For this review, take the finished solid that the model builds, in its own axes (mm). A direction names the side the tool comes from. Round coordinates to 2 decimals unless told otherwise and drop trailing zeros. Loops run counter-clockwise (first coordinate to the right, second up) from the corner with the lowest first, then second, coordinate; pieces in that order, holes last.
```python
from build123d import *

# Parameters (mm, degrees)
F1_DEPTH = 5
F2_T     = -2.5
F3_DEPTH = 25


with BuildPart() as f1:
    # F0 (on Front) → F1 (new body)
    with BuildSketch(Plane.XZ):
        with BuildLine():
            Line((-32.5, -5), (32.5, -5))
            ThreePointArc((32.5, -5), (36.0355339059, -3.5355339059), (37.5, 0))
            ThreePointArc((37.5, 0), (36.0355339059, 3.5355339059), (32.5, 5))
            Line((32.5, 5), (-32.5, 5))
            ThreePointArc((-32.5, 5), (-36.0355339059, 3.5355339059), (-37.5, 0))
            ThreePointArc((-37.5, 0), (-36.0355339059, -3.5355339059), (-32.5, -5))
        make_face()
    extrude(amount=F1_DEPTH)

    # F2
    f2_openings = [f1.faces().sort_by_distance(p)[0] for p in [
        (0, -5, 0),
    ]]
    offset(amount=F2_T, openings=f2_openings)

    # F3 (cut): a face of the model
    f3_faces = [f1.faces().sort_by_distance(p)[0] for p in [
        (0, -2.5, 0),
    ]]
    extrude(f3_faces, amount=-F3_DEPTH, mode=Mode.SUBTRACT)


solid = f1.part
```
(1) For L1, parallel to Z at x = -7.5, y = -1.65; L2, parallel to X at y = -1, z = -1; L3, parallel to X at y = -2.6, z = 2, list the stretches that pass through material, from the lowest coordinate up.
(2) The part is to be moulded in two halves that separate along X. For faces 3 (the flat face through (-1, -5, 3)), 4 (the flat face through (0, -3, 2.5)), say which applies: pulls with the +X half, pulls with the -X half, needs draft (parallel to the pull), parting line crosses it, or undercut.
(3) Add section B-B (x = 15). Give the boundary of the cut face in (y, z), plus the area to 3 significant figures.
(4) Add section C-C (z = 1). Give the boundary of the cut face in (x, y), plus the area to 3 significant figures.
(5) Add section A-A (y = -3.65). Give the boundary of the cut face in (x, z).
(6) For faces 1 (the flat face through (0, -3, -2.5)), 2 (the flat face through (0, -2, 5)), list the 3-axis set-ups (+Z, -Z, +X, -X, +Y, -Y) from which the entire face can be reached by the end or side of a thin tool; tool diameter is ignored.
(7) Add section D-D (z = 4). Give the boundary of the cut face in (x, y).
Outcome:
1. L1: z = -5 to -2.5, 2.5 to 5
1. L2: x = -37.4 to -34.79, 34.79 to 37.4
1. L3: x = -37.08 to -34, 34 to 37.08
2. face 3: needs draft
2. face 4: undercut
3. outline: (-5, -5) - (0, -5) - (0, -2.5) - (-5, -2.5) - close; (-5, 2.5) - (0, 2.5) - (0, 5) - (-5, 5) - close
3. area: 25.0 mm2
4. outline: (-37.4, -5) - (-34.79, -5) - (-34.79, 0) - (-37.4, 0) - close; (34.79, -5) - (37.4, -5) - (37.4, 0) - (34.79, 0) - close
4. area: 26.1 mm2
5. outline: (-32.5, -5) - (32.5, -5) arc R5 ccw to (32.5, 5) - (-32.5, 5) arc R5 ccw to start; hole (-32.5, -2.5) - (32.5, -2.5) arc R2.5 ccw to (32.5, 2.5) - (-32.5, 2.5) arc R2.5 ccw to start
6. face 1: +Y, -Y
6. face 2: +Z, +X, -X, +Y, -Y
7. outline: (-35.5, -5) - (35.5, -5) - (35.5, 0) - (-35.5, 0) - close
